```python
from build123d import *

# Parameters (mm, degrees)
F0_W     = 30
F0_H     = 10
F1_DEPTH = 6
F2_W     = 34
F2_H     = 10
F3_DEPTH = 15
F4_W     = 30
F4_H     = 10
F5_DEPTH = 3


with BuildPart() as f1:
    # F0 (on Top) → F1 (new body)
    with BuildSketch(Plane.XY):
        Rectangle(F0_W, F0_H)
    extrude(amount=F1_DEPTH)

    # F2 (on face) → F3 (join)
    with BuildSketch(Plane.XY.offset(6)):
        Rectangle(F2_W, F2_H)
    extrude(amount=F3_DEPTH)

    # F4 (on face) → F5 (join)
    with BuildSketch(Plane.XY.offset(21)):
        Rectangle(F4_W, F4_H)
    extrude(amount=F5_DEPTH)


solid = f1.part
```
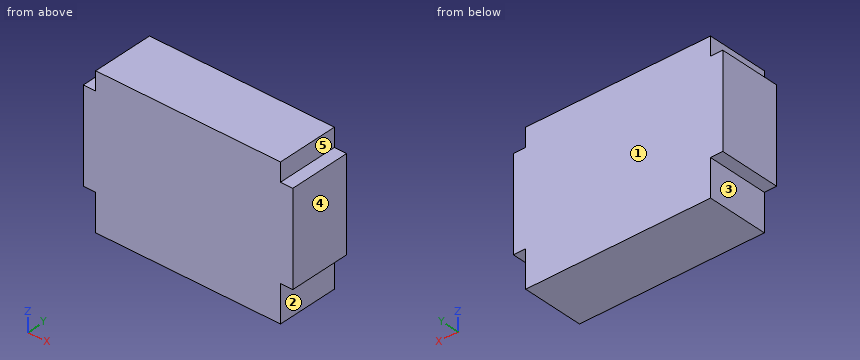
Check sheet for the modelled part. Datum: model origin and axes. Units: mm. Face numbers are marked on the shaded views. A direction names the side the tool comes from. Give positions to 0.01 mm unless a question says otherwise; leave off trailing zeros. Order: outer loops, then holes, each group sorted by start corner. A loop starts at its lowest first (then second) coordinate and runs counter-clockwise, first axis right, second up. Notation, with made-up numbers: M 88,42.25 L 141,42.25 A29 cw 141,78.25 Z; hole C -21.75,75.5 d5. An arc over 180 degrees is marked long. Answer in a Markdown table with one row per item.
1) Gauge pin test, flat ends, axial feed: P1, Ø3, axis at y = 0, z = 2, coming from the +X side; P2, Ø1, axis at x = -16.5, y = 2, coming from the +Z side; P3, Ø1.5, axis at y = 0.5, z = 23, coming from the -X side. Record the tip position at first contact, or that the pin passes through.
Filled sheet:
| item | result |
|---|---|
| P1 | stops at x = 15 |
| P2 | stops at z = 21 |
| P3 | stops at x = -15 |
2) Cross-section at A-A, the plane y = 3.25. Enter the section's corners in (x, z), plus the area to 3 significant figures.
Filled sheet:
| item | result |
|---|---|
| outline | M -17,6 L -15,6 L -15,0 L 15,0 L 15,6 L 17,6 L 17,21 L 15,21 L 15,24 L -15,24 L -15,21 L -17,21 Z |
| area | 780 mm2 |
3) Thickness scan on L1, parallel to X at y = -2, z = 21.25. Record the ranges inside material, lowest first. Write a range as [from, to].
Filled sheet:
| item | result |
|---|---|
| L1 | x = [-15, 15] |
4) Access from +Z, -Z, +X, -X, +Y, -Y to the whole of each face (thin tool, end or side, straight path). Record for the marked faces 1, 2, 3, 4 and 5.
Filled sheet:
| item | result |
|---|---|
| face 1 | +Z, -Z, +X, -X, +Y |
| face 2 | -Z, +X, +Y, -Y |
| face 3 | -Z, -X, +Y, -Y |
| face 4 | +Z, -Z, +X, +Y, -Y |
| face 5 | +Z, +X, +Y, -Y |
5) Cross-section at B-B, the plane z = 3.25. Enter the section's corners in (x, y), plus the area to 3 significant figures.
Filled sheet:
| item | result |
|---|---|
| outline | M -15,-5 L 15,-5 L 15,5 L -15,5 Z |
| area | 300 mm2 |
